Model file for the job. Use its own axes, mm. Face numbers are marked on the shaded views. A direction names the side the tool comes from. Coordinates: 2 decimals unless noted, no trailing zeros. Loops run counter-clockwise (first coordinate to the right, second up) from the corner with the lowest first, then second, coordinate; pieces in that order, holes last. Notation, with made-up numbers: (-30, -11.5) -> (0, -11.5) arc R9 ccw to (0, 5.5) -> close; hole circle Ø6 at (41, 60). An arc over 180 degrees is marked (long way). Use one line per item in the form item = value.
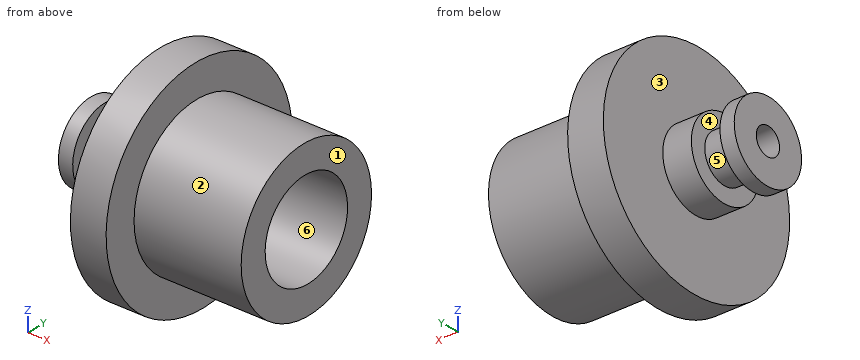
```python
from build123d import *

# Parameters (mm, degrees)
PIPE_TAP_DRILL_FOR_1_8_TAP1_D       = 8.4328
PIPE_TAP_DRILL_FOR_1_8_TAP1_DEPTH   = 9.525
PIPE_TAP_DRILL_FOR_1_8_TAP1_TIP     = 2.533468714
F_3_32_0_09375_DIAMETER_HOLE2_D     = 2.38125
F_3_32_0_09375_DIAMETER_HOLE2_DEPTH = 12.7
F_3_32_0_09375_DIAMETER_HOLE2_TIP   = 0.715399675


with BuildPart() as part:
    # Sketch1 → Revolve1 (revolve)
    with BuildSketch(Plane.XY, mode=Mode.PRIVATE) as revolve1_sk:
        Polygon((6.35, 3.444875), (6.35, 9.525), (9.525, 9.525), (9.525, 6.6675), (19.05, 6.6675), (19.05, 0), (0, 0), (0, 3.444875), (1.27, 3.444875), (1.27, 2.073275), (3.81, 2.073275), (3.81, 3.444875), align=None)
    revolve(revolve1_sk.sketch.rotate(Axis((0, 0, 0), (1, 0, 0)), 90), axis=Axis((0, 0, 0), (1, 0, 0)))

    # Pipe Tap Drill for 1/8 Tap1
    with Locations(Plane(origin=(19.05, 0, 0), x_dir=(0, 0, -1), z_dir=(1, 0, 0))):
        with Locations((0, 0)):
            Hole(PIPE_TAP_DRILL_FOR_1_8_TAP1_D / 2, depth=PIPE_TAP_DRILL_FOR_1_8_TAP1_DEPTH)
            with Locations((0, 0, -(PIPE_TAP_DRILL_FOR_1_8_TAP1_DEPTH + PIPE_TAP_DRILL_FOR_1_8_TAP1_TIP / 2))):  # 118° drill point
                Cone(0, PIPE_TAP_DRILL_FOR_1_8_TAP1_D / 2, PIPE_TAP_DRILL_FOR_1_8_TAP1_TIP, mode=Mode.SUBTRACT)

    # 3/32 (0.09375) Diameter Hole2
    with Locations(Plane.ZY):
        with Locations((0, 0)):
            Hole(F_3_32_0_09375_DIAMETER_HOLE2_D / 2, depth=F_3_32_0_09375_DIAMETER_HOLE2_DEPTH)
            with Locations((0, 0, -(F_3_32_0_09375_DIAMETER_HOLE2_DEPTH + F_3_32_0_09375_DIAMETER_HOLE2_TIP / 2))):  # 118° drill point
                Cone(0, F_3_32_0_09375_DIAMETER_HOLE2_D / 2, F_3_32_0_09375_DIAMETER_HOLE2_TIP, mode=Mode.SUBTRACT)


solid = part.part
```
Q1. Band-saw the part on D-D, the plane y = -5.75. Write the cut outline in (x, z) (3 decimals).
Result:
outline = (6.35, -7.594) -> (9.525, -7.594) -> (9.525, -3.375) -> (19.05, -3.375) -> (19.05, 3.375) -> (9.525, 3.375) -> (9.525, 7.594) -> (6.35, 7.594) -> close
Q2. Wall check: line 1 along Y through (x, z) = (4, 0); line 2 along Y through (x, z) = (16.5, 0); line 3 along X through (y, z) = (0.75, 6.5). Give the ranges that are in metal, low to high.
Result:
line_1 = -3.44 to -1.19, 1.19 to 3.44
line_2 = -6.67 to -4.22, 4.22 to 6.67
line_3 = 6.35 to 19.05
Q3. Mould opens along Y. For the marked faces 4, 5 and 6 say: released by +Y, released by -Y, zero draft, split by the parting line, or undercut.
Result:
face_4 = zero draft
face_5 = split by the parting line
face_6 = undercut
Q4. Pin check, flat tips, straight feed: pin 1 Ø2 at (y, z) = (0.5, 1) entering from -X; pin 2 Ø2 at (y, z) = (0, 0) entering from -X; pin 3 Ø1 at (x, z) = (8.5, 3.5) entering from -Y; pin 4 Ø1 at (x, z) = (16.5, -5) entering from -Y. Stop position of each tip, or through.
Result:
pin_1 = 0
pin_2 = through
pin_3 = -9.04
pin_4 = -4.92
Q5. Which spindle directions (+Z, -Z, +X, -X, +Y, -Y) get a long thin tool onto all of the face, cutting with end or side? Do the marked faces 1, 2 and 3. Say none if no direction does.
Result:
face_1 = +Z, -Z, +X, +Y, -Y
face_2 = +X
face_3 = -X
Q6. Band-saw the part on C-C, the plane x = 7. Write the cut outline in (y, z) (3 decimals).
Result:
outline = circle Ø19.05 at (0, 0); hole circle Ø2.381 at (0, 0)
